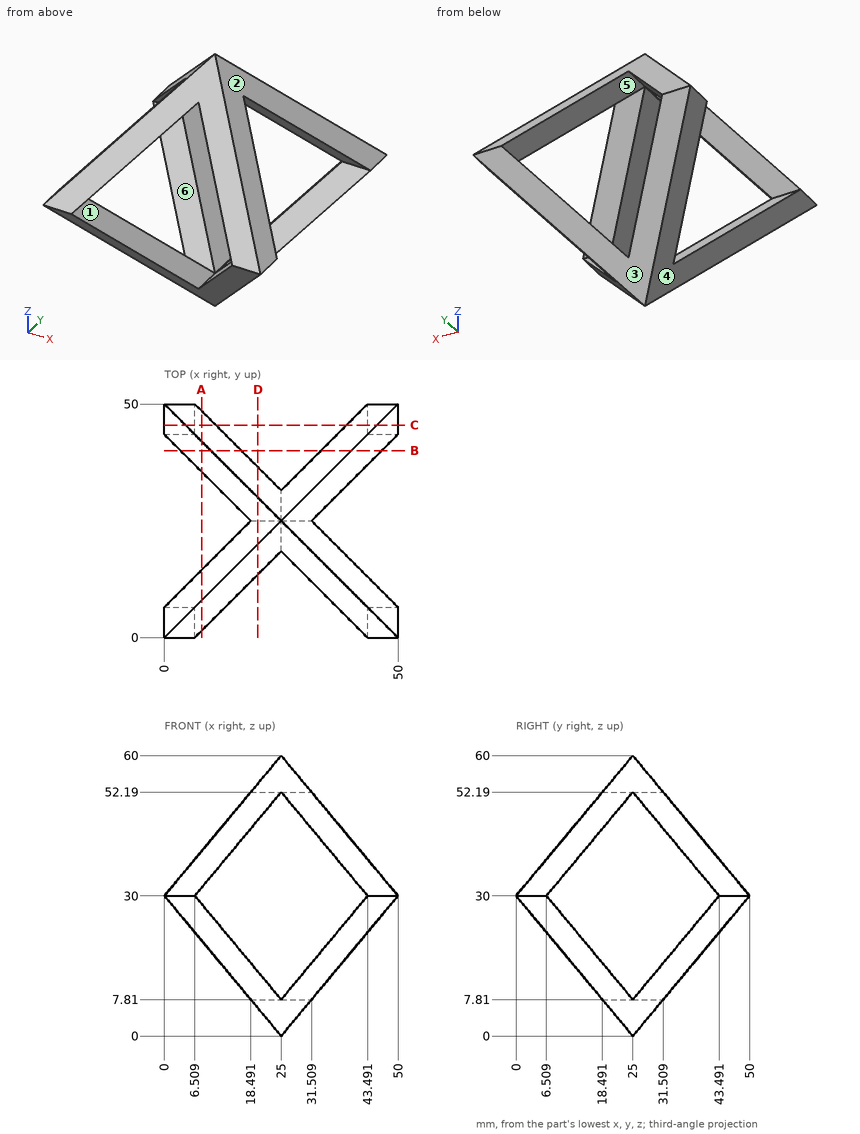
Input: dimensioned drawing with shaded views. Units: mm. Origin: part minimum x, y, z. A direction names the side the tool comes from. Round coordinates to 2 decimals unless told otherwise and drop trailing zeros. Loops run counter-clockwise (first coordinate to the right, second up) from the corner with the lowest first, then second, coordinate; pieces in that order, holes last. Notation, with made-up numbers: (55.25, 67.5) -> (75.25, 67.5) arc R29 cw to (75.25, 88.5) -> close; hole circle Ø2 at (56.5, -12.5). An arc over 180 degrees is marked (long way). Answer as a JSON object with one key per item and string values. Group by question number.
1) Pin query (flat end, axial travel): pin 1 (1 mm diameter, centred on x = 20, z = 43, fed in from +Y); pin 2 (1 mm diameter, centred on x = 30, z = 50.5, fed in from +Y); pin 3 (3 mm diameter, centred on x = 43.5, y = 10.5, fed in from -Z); pin 4 (1 mm diameter, centred on x = 17.5, y = 11.5, fed in from +Z). Return the tip coordinate at first contact, or that it passes through.
2) Draft query along Z for the marked faces 1, 2 and 3. Return one class per face: +Z half, -Z half, draft (parallel to the pull), parting line (faces both ways), or undercut.
3) Section query C-C on y = 45.5. Output: boundary loops of the cut face in (x, z), plus the area to 3 significant figures.
4) Section query B-B on y = 40. Output: boundary loops of the cut face in (x, z).
5) Section query A-A on x = 8. Output: boundary loops of the cut face in (y, z), plus the area to 3 significant figures.
6) Ray query, L1, parallel to Z at x = 8, y = 7; L2, parallel to Z at x = 32.5, y = 20; L3, parallel to X at y = 3, z = 33. Return the intervals inside material, ascending.
7) Section query D-D on x = 20. Output: boundary loops of the cut face in (y, z).
8) Reachability of the marked faces 4, 5 and 6 from +Z, -Z, +X, -X, +Y, -Y: full face, straight path, thin tool, end or side. Return the list, or none.
Reply:
{
 "1": {"pin 1": "passes through", "pin 2": "stops at y = 33.33", "pin 3": "stops at z = 20.4", "pin 4": "stops at z = 44.4"},
 "2": {"face 1": "undercut", "face 2": "+Z half", "face 3": "-Z half"},
 "3": {"outline": "(0, 30) -> (4.5, 24.6) -> (11.01, 24.6) -> (6.51, 30) -> (11.01, 35.4) -> (4.5, 35.4) -> close; (38.99, 24.6) -> (45.5, 24.6) -> (50, 30) -> (45.5, 35.4) -> (38.99, 35.4) -> (43.49, 30) -> close", "area": "141 mm2"},
 "4": {"outline": "(3.49, 25.81) -> (10, 18) -> (16.51, 18) -> (10, 25.81) -> close; (3.49, 34.19) -> (10, 34.19) -> (16.51, 42) -> (10, 42) -> close; (33.49, 18) -> (40, 18) -> (46.51, 25.81) -> (40, 25.81) -> close; (33.49, 42) -> (40, 34.19) -> (46.51, 34.19) -> (40, 42) -> close"},
 "5": {"outline": "(1.49, 28.21) -> (8, 20.4) -> (14.51, 20.4) -> (8, 28.21) -> close; (1.49, 31.79) -> (8, 31.79) -> (14.51, 39.6) -> (8, 39.6) -> close; (35.49, 20.4) -> (42, 20.4) -> (48.51, 28.21) -> (42, 28.21) -> close; (35.49, 39.6) -> (42, 31.79) -> (48.51, 31.79) -> (42, 39.6) -> close", "area": "203 mm2"},
 "6": {"L1": "z = 21.6 to 28.21, 31.79 to 38.4", "L2": "z = 9 to 13.81, 46.19 to 51", "L3": "x = 2.5 to 9.01, 40.99 to 47.5"},
 "7": {"outline": "(13.49, 13.81) -> (20, 6) -> (30, 6) -> (36.51, 13.81) -> (30, 13.81) -> (25, 7.81) -> (20, 13.81) -> close; (13.49, 46.19) -> (20, 46.19) -> (25, 52.19) -> (30, 46.19) -> (36.51, 46.19) -> (30, 54) -> (20, 54) -> close"},
 "8": {"face 4": "-Z, -X, +Y, -Y", "face 5": "+Y, -Y", "face 6": "+X, -X"}
}
